Source: CAD feature listing. Evaluate the final solid. Frame: model axes, mm. Round coordinates to 2 decimals unless told otherwise and drop trailing zeros. Order: outer loops, then holes, each group sorted by start corner. A loop starts at its lowest first (then second) coordinate and runs counter-clockwise, first axis right, second up. Notation, with made-up numbers: (2.25, -7) - (21.25, -7) arc R20 cw to (21.25, 15) - close; hole circle Ø8 at (66, -30). An arc over 180 degrees is marked (long way). Use one line per item in the form item = value. Start each with the question number.
Q1. Cut plane D-D, the plane x = 15. Return the cut outline in (y, z), and give its area (3 significant figures).
Q2. Cut plane A-A, the plane x = 31. Return the cut outline in (y, z), and give its area (3 significant figures).
Q3. Pin query (flat end, axial travel): pin 1 Ø1 at (x, z) = (25, 0.5) entering from -Y; pin 2 Ø0.6 at (y, z) = (1.5, 0.5) entering from +X; pin 3 Ø1 at (x, z) = (64, 1) entering from +Y; pin 4 Ø12 at (x, y) = (40, 7) entering from -Z. Return the tip coordinate at first contact, or that it passes through.
Q4. Ray query, line 1 (Y direction, x = 23, z = 1.9); line 2 (Y direction, x = 67.5, z = 0.8); line 3 (Y direction, x = 18.5, z = 0.6). Return the intervals inside material, ascending. Write a range as [from, to].
Q5. Cut plane C-C, the plane y = 14. Return the cut outline in (x, z), and give its area (3 significant figures).
Q6. Cut plane B-B, the plane z = 1.4. Give the number of separate pieces and of enclosed holes in the cut face, and give its area (3 significant figures).
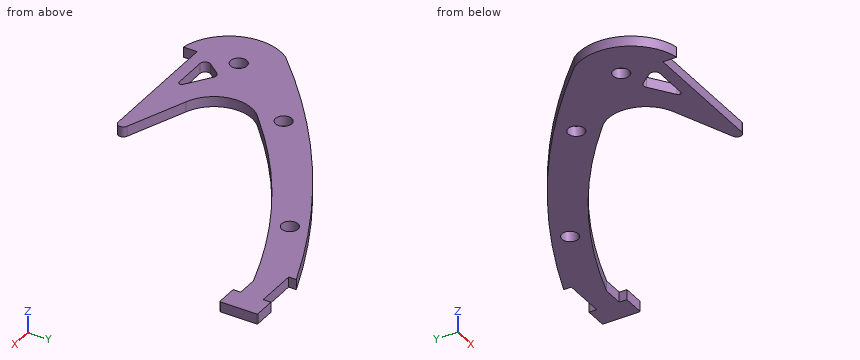
Autodesk Inventor part; units mm, degrees
ref_plane "YZ Plane" through (0, 0, 0) normal (1, 0, 0) x (0, 1, 0)
ref_plane "XZ Plane" through (0, 0, 0) normal (0, 1, 0) x (-1, 0, 0)
ref_plane "XY Plane" through (0, 0, 0) normal (0, 0, 1) x (1, 0, 0)
sketch "Side Part" plane through (0, 0, 0) normal (0, 0, 1) x (1, 0, 0)
  arc A0 (59.2149, 53.2214) -> (1.9677, 16.0747) centre (117.7132, -99.6165) ccw
  arc A1 (63.2649, 47.3171) -> (19.3751, 21.046) centre (99.8299, -63.5681) ccw
  arc A2 (19.3751, 21.046) -> (22.0544, 9.2781) centre (24.9814, 16.1335) ccw
  arc A3 (1.9677, 16.0747) -> (8.356, 0) centre (10.2097, 10.0435) ccw
  circle A4 centre (18.9507, 26.1162) radius 1.6
  circle A5 centre (45.9082, 43.8146) radius 1.6
  line L0 (8.356, 0) -> (8.356, 2.7)
  line L1 (59.2149, 53.2214) -> (59.2149, 51.7214)
  line L2 (59.2149, 51.7214) -> (67.3149, 51.7214)
  line L3 (67.3149, 51.7214) -> (67.3149, 53.2214)
  line L4 (71.631, 46.0171) -> (71.631, 53.0214)
  line L5 (67.3149, 53.2214) -> (71.431, 53.2214)
  arc A6 (71.631, 53.0214) -> (71.431, 53.2214) centre (71.431, 53.0214) ccw
  arc A7 (22.0544, 9.2781) -> (22.0677, 9.2723) centre (22.1405, 9.4586) ccw
  circle A8 centre (7.756, 10.482) radius 1.6
  line L6 (12.2179, 8.9259) -> (10.405, 6.6138)
  arc A9 (10.405, 6.6138) -> (11.1919, 4.9967) centre (11.1919, 5.9967) ccw
  line L7 (11.1919, 4.9967) -> (17.8503, 4.9967)
  line L8 (18.1389, 5.9051) -> (13.582, 9.1255)
  arc A10 (17.8503, 4.9967) -> (18.1389, 5.9051) centre (17.8503, 5.4967) ccw
  arc A11 (13.582, 9.1255) -> (12.2179, 8.9259) centre (13.0048, 8.3088) ccw
  line L9 (8.356, 2.7) -> (33.5768, 2.7)
  arc A12 (33.5768, 2.7) -> (33.9408, 4.6314) centre (33.5768, 3.7) ccw
  line L10 (33.9408, 4.6314) -> (22.0677, 9.2723)
  line L11 (67.3149, 45.8171) -> (67.3149, 47.3171)
  line L12 (67.3149, 45.8171) -> (71.431, 45.8171)
  arc A13 (71.431, 45.8171) -> (71.631, 46.0171) centre (71.431, 46.0171) ccw
  line L13 (63.2649, 47.3171) -> (67.3149, 47.3171)
  point P0 (38.6259, 23.714)
sketch "Sketch1" plane through (0, 0, 0) normal (0, 0, 1) x (1, 0, 0)
  circle A0 centre (45.9082, 43.8146) radius 1.6
  circle A1 centre (18.9507, 26.1162) radius 1.6
  circle A2 centre (7.756, 10.482) radius 1.6
  arc A3 (10.405, 6.6138) -> (11.1919, 4.9967) centre (11.1919, 5.9967) ccw
  arc A4 (13.582, 9.1255) -> (12.2179, 8.9259) centre (13.0048, 8.3088) ccw
  arc A5 (17.8503, 4.9967) -> (18.1389, 5.9051) centre (17.8503, 5.4967) ccw
  arc A6 (20.4302, 22.0369) -> (22.4669, 9.1163) centre (24.9814, 16.1335) ccw
  arc A7 (33.5768, 2.7) -> (33.9408, 4.6314) centre (33.5768, 3.7) ccw
  arc A8 (4.3433, 18.4037) -> (8.356, 0) centre (10.2097, 10.0435) ccw
  line L0 (8.356, 0) -> (8.356, 2.7)
  line L1 (8.356, 2.7) -> (33.5768, 2.7)
  line L2 (33.9408, 4.6314) -> (22.4669, 9.1163)
  line L3 (18.1389, 5.9051) -> (13.582, 9.1255)
  line L4 (11.1919, 4.9967) -> (17.8503, 4.9967)
  line L5 (12.2179, 8.9259) -> (10.405, 6.6138)
  arc A9 (59.2149, 53.2214) -> (1.9677, 16.0747) centre (117.7132, -99.6165) ccw
  arc A10 (63.2649, 47.3171) -> (19.3751, 21.046) centre (99.8299, -63.5681) ccw
  line L6 (59.2149, 53.2214) -> (59.2149, 51.7214)
  line L7 (59.2149, 51.7214) -> (67.3149, 51.7214)
  line L8 (67.3149, 51.7214) -> (67.3149, 53.2214)
  arc A11 (71.631, 53.0214) -> (71.431, 53.2214) centre (71.431, 53.0214) ccw
  arc A12 (71.431, 45.8171) -> (71.631, 46.0171) centre (71.431, 46.0171) ccw
  line L9 (67.3149, 53.2214) -> (71.431, 53.2214)
  line L10 (71.631, 53.0214) -> (71.631, 46.0171)
  line L11 (71.431, 45.8171) -> (67.3149, 45.8171)
  line L12 (67.3149, 45.8171) -> (67.3149, 47.3171)
  line L13 (67.3149, 47.3171) -> (63.2649, 47.3171)
  arc A13 (59.2149, 53.2214) -> (1.9677, 16.0747) centre (117.7132, -99.6165) ccw
  arc A14 (63.2649, 47.3171) -> (19.3751, 21.046) centre (99.8299, -63.5681) ccw
  arc A15 (19.3751, 21.046) -> (22.0544, 9.2781) centre (24.9814, 16.1335) ccw
  arc A16 (1.9677, 16.0747) -> (8.356, 0) centre (10.2097, 10.0435) ccw
  circle A17 centre (18.9507, 26.1162) radius 1.6
  circle A18 centre (45.9082, 43.8146) radius 1.6
  line L14 (8.356, 0) -> (8.356, 2.7)
  line L15 (59.2149, 53.2214) -> (59.2149, 51.7214)
  line L16 (59.2149, 51.7214) -> (67.3149, 51.7214)
  line L17 (67.3149, 51.7214) -> (67.3149, 53.2214)
  line L18 (71.631, 46.0171) -> (71.631, 53.0214)
  line L19 (67.3149, 53.2214) -> (71.431, 53.2214)
  arc A19 (71.631, 53.0214) -> (71.431, 53.2214) centre (71.431, 53.0214) ccw
  arc A20 (22.0544, 9.2781) -> (22.0677, 9.2723) centre (22.1405, 9.4586) ccw
  circle A21 centre (7.756, 10.482) radius 1.6
  line L20 (12.2179, 8.9259) -> (10.405, 6.6138)
  arc A22 (10.405, 6.6138) -> (11.1919, 4.9967) centre (11.1919, 5.9967) ccw
  line L21 (11.1919, 4.9967) -> (17.8503, 4.9967)
  line L22 (18.1389, 5.9051) -> (13.582, 9.1255)
  arc A23 (17.8503, 4.9967) -> (18.1389, 5.9051) centre (17.8503, 5.4967) ccw
  arc A24 (13.582, 9.1255) -> (12.2179, 8.9259) centre (13.0048, 8.3088) ccw
  line L23 (8.356, 2.7) -> (33.5768, 2.7)
  arc A25 (33.5768, 2.7) -> (33.9408, 4.6314) centre (33.5768, 3.7) ccw
  line L24 (33.9408, 4.6314) -> (22.0677, 9.2723)
  line L25 (67.3149, 45.8171) -> (67.3149, 47.3171)
  line L26 (67.3149, 45.8171) -> (71.431, 45.8171)
  arc A26 (71.431, 45.8171) -> (71.631, 46.0171) centre (71.431, 46.0171) ccw
  line L27 (63.2649, 47.3171) -> (67.3149, 47.3171)
  point P0 (0, 0)
extrude "Extrusion1" add sketch "Sketch1" along normal blind 2 contours A6 L2 A7 L1 L0 A8 A9 L6 L7 L8 L9 A11 L10 A12 L11 L12 L13 A10
properties part number "Side_Part"
Completed:
q1.outline = (2.7, 0) - (5, 0) - (5, 2) - (2.7, 2) - close; (8.12, 0) - (27.79, 0) - (27.79, 2) - (8.12, 2) - close
q1.area = 43.9 mm2
q2.outline = (2.7, 0) - (5.78, 0) - (5.78, 2) - (2.7, 2) - close; (30.75, 0) - (39.17, 0) - (39.17, 2) - (30.75, 2) - close
q2.area = 23.0 mm2
q3.pin_1 = 2.7
q3.pin_2 = 8.36
q3.pin_3 = 51.72
q3.pin_4 = through
q4.line_1 = [2.7, 8.91], [24.35, 33.84]
q4.line_2 = [45.82, 53.22]
q4.line_3 = [2.7, 12.45], [19.82, 24.58], [27.65, 30.53]
q5.outline = (0.79, 0) - (17.84, 0) - (17.84, 2) - (0.79, 2) - close
q5.area = 34.1 mm2
q6.separate_pieces = 1
q6.enclosed_holes = 4
q6.area = 799 mm2
